Can you work these out from the model? Positions are in its coordinate system, mm. A direction names the side the tool comes from. Coordinates: 2 decimals unless noted, no trailing zeros. Order: outer loops, then holes, each group sorted by start corner. A loop starts at its lowest first (then second) coordinate and runs counter-clockwise, first axis right, second up. Notation, with made-up numbers: M 47,82 L 63,82 A11 ccw 63,93 Z; hole C 18,16.25 d11. An arc over 180 degrees is marked long. Answer as a JSON object with one key per item and string values.
from build123d import *

# Parameters (mm, degrees)
ESTRUSIONE_ESTRUSIONE1_DEPTH   = 105
ESTRUSIONE_ESTRUSIONE1_2_DEPTH = 105
SCHIZZO2_W                     = 28.749445424
SCHIZZO2_H                     = 105
ESTRUSIONE_ESTRUSIONE2_DEPTH   = 10
ESTRUSIONE_ESTRUSIONE3_DEPTH   = 35.85
SCHIZZO4_W                     = 30
SCHIZZO4_H                     = 71.7
ESTRUSIONE_ESTRUSIONE4_DEPTH   = 130
SCHIZZO5_W                     = 125.014718626
SCHIZZO5_H                     = 71.7
ESTRUSIONE_ESTRUSIONE5_DEPTH   = 20
SMUSSO1_SIZE                   = 20


with BuildPart() as part:
    # Schizzo1 → Estrusione-Estrusione1 (new body)
    with BuildSketch(Plane.XY):
        with BuildLine():
            ThreePointArc((14.374722712, 4.285714286), (0, 15), (-14.374722712, 4.285714286))
            Line((-14.374722712, 4.285714286), (14.374722712, 4.285714286))
        make_face()
    extrude(amount=-ESTRUSIONE_ESTRUSIONE1_DEPTH)



with BuildPart() as body_2:
    # Schizzo1 → Estrusione-Estrusione1 2 (new body)
    with BuildSketch(Plane.XY):
        with BuildLine():
            Line((75.625277288, 4.285714286), (104.374722712, 4.285714286))
            ThreePointArc((104.374722712, 4.285714286), (90, 15), (75.625277288, 4.285714286))
        make_face()
    extrude(amount=-ESTRUSIONE_ESTRUSIONE1_2_DEPTH)


with BuildPart() as part_1:
    add(part.part)

    add(body_2.part)  # Estrusione-Estrusione2 merges body 2
    # Schizzo2 → Estrusione-Estrusione2 (add)
    with BuildSketch(Plane.XZ.offset(-4.285714286)):
        with Locations((0, -52.5)):
            Rectangle(SCHIZZO2_W, SCHIZZO2_H)
        with Locations((90, -52.5)):
            Rectangle(SCHIZZO2_W, SCHIZZO2_H)
    extrude(amount=ESTRUSIONE_ESTRUSIONE2_DEPTH)

    # Schizzo3 → Estrusione-Estrusione3 (add, symmetric)
    with BuildSketch(Plane.XY):
        with BuildLine():
            Line((-14.374722712, -5.714285714), (104.374722712, -5.714285714))
            Line((104.374722712, -5.714285714), (104.374722712, 4.285714286))
            ThreePointArc((104.374722712, 4.285714286), (98.96421457, 12.026755886), (90, 15))
            Line((90, 15), (0, 15))
            ThreePointArc((0, 15), (-8.96421457, 12.026755886), (-14.374722712, 4.285714286))
            Line((-14.374722712, 4.285714286), (-14.374722712, -5.714285714))
        make_face()
    extrude(amount=ESTRUSIONE_ESTRUSIONE3_DEPTH, both=True)

    # Schizzo4 → Estrusione-Estrusione4 (add)
    with BuildSketch(Plane(origin=(0, 15, 0), x_dir=(1, 0, 0), z_dir=(0, 1, 0))):
        with Locations((45, 0)):
            Rectangle(SCHIZZO4_W, SCHIZZO4_H)
    extrude(amount=ESTRUSIONE_ESTRUSIONE4_DEPTH)

    # Schizzo5 → Estrusione-Estrusione5 (add)
    with BuildSketch(Plane(origin=(0, 145, -145), x_dir=(1, 0, 0), z_dir=(0, -1, 0))):
        with Locations((45, 145)):
            Rectangle(SCHIZZO5_W, SCHIZZO5_H)
        with BuildLine():
            ThreePointArc((97, 156.85), (105, 164.85), (97, 172.85))
            ThreePointArc((97, 172.85), (89, 164.85), (97, 156.85))
        make_face(mode=Mode.SUBTRACT)
        with BuildLine():
            ThreePointArc((97, 127.85), (89, 119.85), (97, 111.85))
            ThreePointArc((97, 111.85), (105, 119.85), (97, 127.85))
        make_face(mode=Mode.SUBTRACT)
        with BuildLine():
            ThreePointArc((-7, 127.85), (-15, 119.85), (-7, 111.85))
            ThreePointArc((-7, 111.85), (1, 119.85), (-7, 127.85))
        make_face(mode=Mode.SUBTRACT)
        with BuildLine():
            ThreePointArc((-7, 156.85), (1, 164.85), (-7, 172.85))
            ThreePointArc((-7, 172.85), (-15, 164.85), (-7, 156.85))
        make_face(mode=Mode.SUBTRACT)
    extrude(amount=-ESTRUSIONE_ESTRUSIONE5_DEPTH)

    # Smusso1
    smusso1_edges = [part_1.edges().sort_by_distance(p)[0] for p in [
        (30, 15, 0),
        (60, 15, 0),
        (30, 145, 0),
        (60, 145, 0),
    ]]
    chamfer(smusso1_edges, length=SMUSSO1_SIZE)


solid = part_1.part
Item 1: I want a section at B-B, the plane x = 24.5. Write out the boundary of the cut face in (y, z).
Answers follow:
{"outline": "M -5.71,-35.85 L 29.5,-35.85 L 29.5,35.85 L -5.71,35.85 Z; M 130.5,-35.85 L 165,-35.85 L 165,35.85 L 130.5,35.85 Z"}
Item 2: I want a section at A-A, the plane z = -82.5. Write out the boundary of the cut face in (x, y).
Answers follow:
{"outline": "M -14.37,-5.71 L 14.37,-5.71 L 14.37,4.29 A15 ccw -14.37,4.29 Z; M 75.63,-5.71 L 104.37,-5.71 L 104.37,4.29 A15 ccw 75.63,4.29 Z"}
Item 3: I'm going to push flat-ended pins straight in: pin 1 (3 mm diameter, centred on y = 0.5, z = -43.5, fed in from +X); pin 2 (5 mm diameter, centred on x = 25, y = 142, fed in from -Z); pin 3 (8 mm diameter, centred on y = -2, z = -10, fed in from -X). Where does each tip first touch, or does it pass through?
Answers follow:
{"pin 1": "stops at x = 104.37", "pin 2": "stops at z = -35.85", "pin 3": "stops at x = -14.37"}
Item 4: Which directions (+Z, -Z, +X, -X, +Y, -Y) give clear straight access to the entire face, cutting with the end or side of a thin tool? Please do faces 4 (the cylindrical face through (-3.95, 14.47, -49.24)), 5 (the cylindrical face through (-2.132, 154.86, 13.501)), 6 (the flat face through (75.625, -1, -71)).
Answers follow:
{"face 4": "-Z", "face 5": "+Y", "face 6": "-Z, +Y, -Y"}
Item 5: If we mould it in two halves opening along X, with no side actions, what happens to faces 1 (the flat face through (20, 135, 1)), 2 (the flat face through (0, 2, -105)), 3 (the cylindrical face through (89.9, 154.86, -28.84))? For each: pulls with the +X half, pulls with the -X half, needs draft (parallel to the pull), parting line crosses it, or undercut.
Answers follow:
{"face 1": "pulls with the -X half", "face 2": "needs draft", "face 3": "undercut"}
Item 6: Please list where these lines run through material, in increasing order: line 1 (X direction, y = 151, z = 19.85); line 2 (Y direction, x = 85, z = -3); line 3 (Z direction, x = 44, y = 18).
Answers follow:
{"line 1": "x = -17.51 to -15, 1 to 89, 105 to 107.51", "line 2": "y = -5.71 to 15, 145 to 165", "line 3": "z = -35.85 to 35.85"}
Item 7: I want a section at D-D, the plane y = 12. Write out the boundary of the cut face in (x, z).
Answers follow:
{"outline": "M -9,-105 L 9,-105 L 9,-35.85 L 81,-35.85 L 81,-105 L 99,-105 L 99,35.85 L -9,35.85 Z"}
Item 8: I want a section at C-C, the plane z = -25.15. Write out the boundary of the cut face in (x, y).
Answers follow:
{"outline": "M -17.51,145 L -15,145 L -15,165 L -17.51,165 Z; M -14.37,-5.71 L 104.37,-5.71 L 104.37,4.29 A15 ccw 90,15 L 80,15 L 60,35 L 60,125 L 80,145 L 89,145 L 89,165 L 1,165 L 1,145 L 10,145 L 30,125 L 30,35 L 10,15 L 0,15 A15 ccw -14.37,4.29 Z; M 105,145 L 107.51,145 L 107.51,165 L 105,165 Z"}
